The figure shows three views and two pictorial views of one solid part (mm, origin at its lowest corner). Answer the questions. Coordinates: 2 decimals unless noted, no trailing zeros. Order: outer loops, then holes, each group sorted by start corner. A loop starts at its lowest first (then second) coordinate and runs counter-clockwise, first axis right, second up. Notation, with made-up numbers: (25.25, 67) -> (56.25, 67) arc R20 ccw to (56.25, 85) -> close; hole circle Ø2 at (-24, 57). An arc over 180 degrees is marked (long way). Use one line per item in the form item = value.
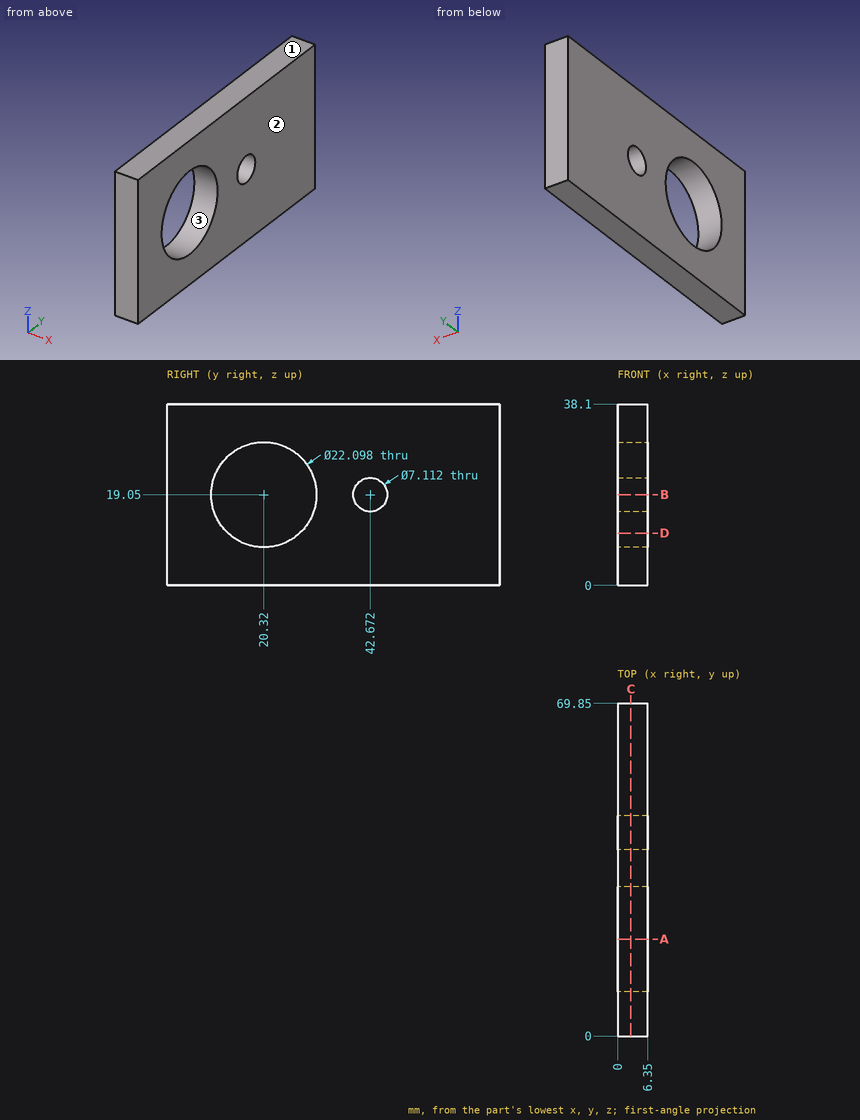
(1) The mould has two halves that part along Z. Classify the marked faces 1, 2 and 3: released by +Z, released by -Z, zero draft, split by the parting line, or undercut.
Data:
face_1 = released by +Z
face_2 = zero draft
face_3 = undercut
(2) Straight lines are drawn through the part: line 1 along Y through (x, z) = (4.75, 19.05); line 2 along Y through (x, z) = (4, 17); line 3 along Z through (x, y) = (2.5, 20.5). For each, find the intervals that lie inside material, in ascending order.
Data:
line_1 = 0 to 9.27, 31.37 to 39.12, 46.23 to 69.85
line_2 = 0 to 9.46, 31.18 to 39.77, 45.58 to 69.85
line_3 = 0 to 8, 30.1 to 38.1
(3) Section B-B on z = 19.05 is taken. Write down the section's boundary in (x, y).
Data:
outline = (0, 0) -> (6.35, 0) -> (6.35, 9.27) -> (0, 9.27) -> close; (0, 31.37) -> (6.35, 31.37) -> (6.35, 39.12) -> (0, 39.12) -> close; (0, 46.23) -> (6.35, 46.23) -> (6.35, 69.85) -> (0, 69.85) -> close
(4) Section C-C on x = 2.75 is taken. Write down the section's boundary in (y, z), plus the area to 3 significant figures.
Data:
outline = (0, 0) -> (69.85, 0) -> (69.85, 38.1) -> (0, 38.1) -> close; hole circle Ø22.1 at (20.32, 19.05); hole circle Ø7.11 at (42.67, 19.05)
area = 2,240 mm²
(5) This flat-tipped pin is pushed along its axis until it touches: P1, Ø17.5, axis at y = 20.32, z = 19.05, coming from the -X side. Where does it stop, or does it pass through?
Data:
P1 = through
(6) Section D-D on z = 11 is taken. Write down the section's boundary in (x, y), plus the area to 3 significant figures.
Data:
outline = (0, 0) -> (6.35, 0) -> (6.35, 12.75) -> (0, 12.75) -> close; (0, 27.89) -> (6.35, 27.89) -> (6.35, 69.85) -> (0, 69.85) -> close
area = 347 mm²
(7) Section A-A on y = 20.32 is taken. Write down the section's boundary in (x, z), plus the area to 3 significant figures.
Data:
outline = (0, 0) -> (6.35, 0) -> (6.35, 8) -> (0, 8) -> close; (0, 30.1) -> (6.35, 30.1) -> (6.35, 38.1) -> (0, 38.1) -> close
area = 102 mm²
